The listing builds one solid part. Answer for the finished solid, in the listing's coordinates (mm). Give positions to 0.01 mm unless a question says otherwise; leave off trailing zeros.
Item 1: The mould has two halves that part along X. Classify faces 1 (the face through (-39, 0, 6)), 2 (the face through (-1.528, -4.944, -51.222)), 3 (the face through (-74.686, -4.944, 60.891)), 4 (the face through (-38, -9.5, -45)): pulls with the +X half, pulls with the -X half, needs draft (parallel to the pull), parting line crosses it, or undercut.
Item 2: Consider line 1 along Z through (x, y) = (-4, -4.75); line 2 along Z through (x, y) = (-18, -9.5); line 3 along X through (y, z) = (-0.75, 28). Determine where each line is inside the solid, lowest interval first.
Item 3: This flat-tipped pin is pushed along its axis until it touches: pin 1 Ø8 at (x, z) = (-36, -43.5) entering from -Y. Where does it stop, or does it pass through?
from build123d import *

# Parameters (mm, degrees)
F0_R     = 5.4921588255
F1_DEPTH = 10
F0_R_2   = 4.8647477
F2_DEPTH = 10
F3_SIZE  = 0.5
F4_DEPTH = 9.5
F5_R     = 1


with BuildPart() as f1:
    # F0 (on Front) → F1 (new body)
    with BuildSketch(Plane.XZ):
        with BuildLine():
            Line((-5.08, 62.3396973443), (-71.1331922889, 62.3396973443))
            ThreePointArc((-71.1331922889, 62.3396973443), (-74.7252947373, 60.8517997927), (-76.2131922889, 57.2596973443))
            Line((-76.2131922889, 57.2596973443), (-76.2131922889, -47.5904377484))
            ThreePointArc((-76.2131922889, -47.5904377484), (-74.7252947373, -51.1825401969), (-71.1331922889, -52.6704377484))
            Line((-71.1331922889, -52.6704377484), (-5.08, -52.6704377484))
            ThreePointArc((-5.08, -52.6704377484), (-1.4878975516, -51.1825401969), (0, -47.5904377484))
            Line((0, -47.5904377484), (0, 57.2596973443))
            ThreePointArc((0, 57.2596973443), (-1.4878975516, 60.8517997927), (-5.08, 62.3396973443))
        make_face()
        with Locations((-38.1065961444, -45.075263828)):
            Circle(F0_R, mode=Mode.SUBTRACT)
        with BuildLine():
            ThreePointArc((-68.5931922889, 44.5596973443), (-67.8492435131, 46.3557485685), (-66.0531922889, 47.0996973443))
            Line((-66.0531922889, 47.0996973443), (-10.16, 47.0996973443))
            ThreePointArc((-10.16, 47.0996973443), (-8.3639487758, 46.3557485685), (-7.62, 44.5596973443))
            Line((-7.62, 44.5596973443), (-7.62, -34.8904377484))
            ThreePointArc((-7.62, -34.8904377484), (-8.3639487758, -36.6864889726), (-10.16, -37.4304377484))
            Line((-10.16, -37.4304377484), (-66.0531922889, -37.4304377484))
            ThreePointArc((-66.0531922889, -37.4304377484), (-67.8492435131, -36.6864889726), (-68.5931922889, -34.8904377484))
            Line((-68.5931922889, -34.8904377484), (-68.5931922889, 44.5596973443))
        make_face(mode=Mode.SUBTRACT)
        with BuildLine():
            Line((-10.16, 47.0996973443), (-66.0531922889, 47.0996973443))
            ThreePointArc((-66.0531922889, 47.0996973443), (-67.8492435131, 46.3557485685), (-68.5931922889, 44.5596973443))
            Line((-68.5931922889, 44.5596973443), (-68.5931922889, -34.8904377484))
            ThreePointArc((-68.5931922889, -34.8904377484), (-67.8492435131, -36.6864889726), (-66.0531922889, -37.4304377484))
            Line((-66.0531922889, -37.4304377484), (-10.16, -37.4304377484))
            ThreePointArc((-10.16, -37.4304377484), (-8.3639487758, -36.6864889726), (-7.62, -34.8904377484))
            Line((-7.62, -34.8904377484), (-7.62, 44.5596973443))
            ThreePointArc((-7.62, 44.5596973443), (-8.3639487758, 46.3557485685), (-10.16, 47.0996973443))
        make_face()
    extrude(amount=F1_DEPTH)

    # F0 (on Front) → F2 (join)
    with BuildSketch(Plane.XZ):
        with Locations((-38.1065961444, -45.075263828)):
            Circle(F0_R)
        with Locations((-38.1065961444, -45.075263828)):
            Circle(F0_R_2, mode=Mode.SUBTRACT)
    extrude(amount=F2_DEPTH)

    # F3
    f3_edges = [f1.edges().sort_by_distance(p)[0] for p in [
        (-42.971344, -10, -45.075264),
    ]]
    chamfer(f3_edges, length=F3_SIZE)

    # F0 (on Front) → F4 (join)
    with BuildSketch(Plane.XZ):
        with Locations((-38.1065961444, -45.075263828)):
            Circle(F0_R_2)
    extrude(amount=F4_DEPTH)

    # F5
    f5_edges = [f1.edges().sort_by_distance(p)[0] for p in [
        (-76.213192, -10, 4.83463),
        (-74.725295, 0, 60.8518),
        (-76.213192, -5, 57.259697),
        (-76.213192, -5, -47.590438),
        (-76.213192, 0, 4.83463),
        (-71.133192, -5, 62.339697),
        (-71.133192, -5, -52.670438),
        (-74.725295, 0, -51.18254),
        (-38.106596, 0, -52.670438),
        (-38.106596, -10, -52.670438),
        (0, -5, -47.590438),
        (-5.08, -5, -52.670438),
        (0, -10, 4.83463),
        (0, 0, 4.83463),
    ]]
    fillet(f5_edges, radius=F5_R)


solid = f1.part
Worked answers:
1. face 1: needs draft
1. face 2: pulls with the +X half
1. face 3: pulls with the -X half
1. face 4: undercut
2. line 1: z = -52.55 to 62.22
2. line 2: z = -52.54 to 62.21
2. line 3: x = -76.18 to -0.03
3. pin 1: stops at y = -10
